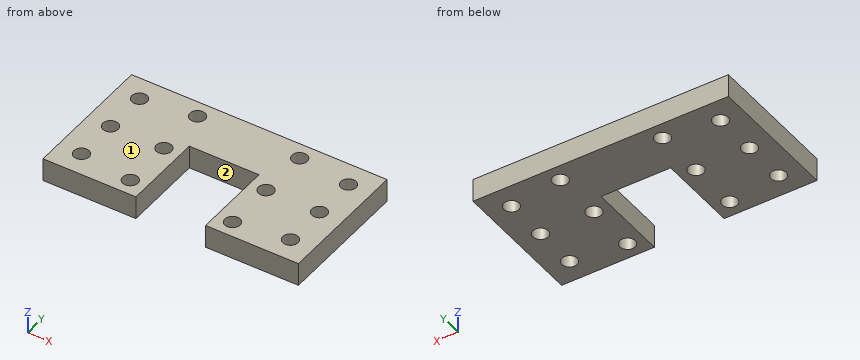
from build123d import *

# Parameters (mm, degrees)
BOSS_EXTRUDE1_DEPTH = 10
M6_CLEARANCE_HOLE_D = 6.6


with BuildPart() as part:
    # Sketch1 → Boss-Extrude1 (new body)
    with BuildSketch(Plane.XY):
        Polygon((55, 0), (15, 0), (15, 35), (-15, 35), (-15, 0), (-55, 0), (-55, 58), (55, 58), align=None)
    extrude(amount=BOSS_EXTRUDE1_DEPTH)

    # M6 Clearance Hole (through all)
    with Locations(Plane(origin=(559.845790405, 1460.886073068, 10), x_dir=(-1, 0, 0), z_dir=(0, 0, 1))):
        with Locations((514.845790405, 1450.886073068), (514.845790405, 1412.886073068), (537.845790405, 1453.886073068), (537.845790405, 1409.886073068), (581.845790405, 1453.886073068), (581.845790405, 1409.886073068), (604.845790405, 1450.886073068), (604.845790405, 1412.886073068), (514.845790405, 897.471608895), (537.845790405, 897.471608895), (581.845790405, 897.471608895), (604.845790405, 897.471608895), (394.752371414, 1482.156083565), (514.845790405, 1431.886073068), (537.845790405, 1431.886073068), (581.845790405, 1431.886073068), (604.845790405, 1431.886073068)):
            Hole(M6_CLEARANCE_HOLE_D / 2)


solid = part.part
Here's how the part is built. I have some questions about the finished solid (model axes, mm). Face numbers are marked on the shaded views. A direction names the side the tool comes from. Round coordinates to 2 decimals unless told otherwise and drop trailing zeros. Write each loop counter-clockwise with the first axis right and the second up, starting at its lowest first coordinate (ties: lowest second). Pieces come first, ordered by that corner, then holes.
1. Suppose I cut it at C-C (z = 3.25). State how many separate pieces and enclosed holes the cut face has, and give its area (3 significant figures).
2. Suppose I cut it at A-A (x = 45). List the corners of the cut face in (y, z) for me, and give its area (3 significant figures).
3. I need wall thicknesses on L1, parallel to Y at x = 22, z = 5.25; L2, parallel to X at y = 29, z = 4; L3, parallel to Y at x = -45, z = 7.75. Which ranges of each line are inside material? Lowest first, please.
4. Suppose I cut it at D-D (x = 12.5). List the corners of the cut face in (y, z) for me, and give its area (3 significant figures).
5. For the marked faces 1 and 2, which set-ups out of +Z, -Z, +X, -X, +Y, -Y let a thin tool reach every point of the face, with its end or its side?
6. Suppose I cut it at B-B (y = 20.5). List the corners of the cut face in (x, z) for me, and give its area (3 significant figures).
7. Will these pins go through, and if not, where does the flat tip stop? pin 1 Ø5 at (x, y) = (23, 20) entering from -Z; pin 2 Ø4 at (x, y) = (-45, 48) entering from +Z.
Answer sheet:
1. separate pieces: 1
1. enclosed holes: 12
1. area: 4,920 mm2
2. outline: (0, 0) - (6.7, 0) - (6.7, 10) - (0, 10) - close; (13.3, 0) - (25.7, 0) - (25.7, 10) - (13.3, 10) - close; (32.3, 0) - (44.7, 0) - (44.7, 10) - (32.3, 10) - close; (51.3, 0) - (58, 0) - (58, 10) - (51.3, 10) - close
2. area: 382 mm2
3. L1: y = 0 to 3.7, 10.3 to 25.7, 32.3 to 47.7, 54.3 to 58
3. L2: x = -55 to -48.3, -41.7 to -25.3, -18.7 to -15, 15 to 18.7, 25.3 to 41.7, 48.3 to 55
3. L3: y = 0 to 6.7, 13.3 to 25.7, 32.3 to 44.7, 51.3 to 58
4. outline: (35, 0) - (58, 0) - (58, 10) - (35, 10) - close
4. area: 230 mm2
5. face 1: +Z, +X, -X, +Y, -Y
5. face 2: +Z, -Z, -Y
6. outline: (-55, 0) - (-15, 0) - (-15, 10) - (-55, 10) - close; (15, 0) - (55, 0) - (55, 10) - (15, 10) - close
6. area: 800 mm2
7. pin 1: stops at z = 0
7. pin 2: passes through
